from build123d import *

# Parameters (mm, degrees)
SURFACE_EXTRUDE1_1_DEPTH = 1200
THICKEN1_T1              = 3
BOSS_EXTRUDE1_REACH      = 1246.822
SKETCH2_W                = 29.7
SKETCH2_H                = 2


with BuildPart() as body_1:
    # Surface-Extrude1: a surface, the sketch's curves swept straight by 1200 mm
    with BuildLine(Plane.XY, mode=Mode.PRIVATE) as surface_extrude1_1_path:
        Line((-30, 329.67), (-30, 130.766968306))
        ThreePointArc((-30, 130.766968306), (-22.403830344, 63.684928981), (0, 0))
    surface_extrude1_1 = Shell.extrude(surface_extrude1_1_path.wire(), (0 * SURFACE_EXTRUDE1_1_DEPTH, 0 * SURFACE_EXTRUDE1_1_DEPTH, 1 * SURFACE_EXTRUDE1_1_DEPTH))
    add(Solid.thicken(surface_extrude1_1, THICKEN1_T1))

    # Sketch2 → Boss-Extrude1 (add, up to next)
    with BuildSketch(Plane(origin=(0, 329.67, 0), x_dir=(1, 0, 0), z_dir=(0, 1, 0)), mode=Mode.PRIVATE) as boss_extrude1_sk1:
        with Locations((-12.15, -1175)):
            Rectangle(SKETCH2_W, SKETCH2_H)
    boss_extrude1_tool1 = extrude(boss_extrude1_sk1.sketch, amount=-BOSS_EXTRUDE1_REACH, mode=Mode.PRIVATE) - body_1.part
    # Sketch2 → Boss-Extrude1 (add, up to next)
    with BuildSketch(Plane(origin=(0, 329.67, 0), x_dir=(1, 0, 0), z_dir=(0, 1, 0)), mode=Mode.PRIVATE) as boss_extrude1_sk2:
        with Locations((-12.15, -600)):
            Rectangle(SKETCH2_W, SKETCH2_H)
    boss_extrude1_tool2 = extrude(boss_extrude1_sk2.sketch, amount=-BOSS_EXTRUDE1_REACH, mode=Mode.PRIVATE) - body_1.part
    # Sketch2 → Boss-Extrude1 (add, up to next)
    with BuildSketch(Plane(origin=(0, 329.67, 0), x_dir=(1, 0, 0), z_dir=(0, 1, 0)), mode=Mode.PRIVATE) as boss_extrude1_sk3:
        with Locations((-12.15, -25)):
            Rectangle(SKETCH2_W, SKETCH2_H)
    boss_extrude1_tool3 = extrude(boss_extrude1_sk3.sketch, amount=-BOSS_EXTRUDE1_REACH, mode=Mode.PRIVATE) - body_1.part
    add(boss_extrude1_tool1.solids().sort_by_distance((-12.15, 329.67, 1175))[0])
    add(boss_extrude1_tool2.solids().sort_by_distance((-12.15, 329.67, 600))[0])
    add(boss_extrude1_tool3.solids().sort_by_distance((-12.15, 329.67, 25))[0])


solid = body_1.part
Could you check a few things on this model? Use its own coordinates, in mm. A direction names the side the tool comes from. Coordinates: 2 decimals unless noted, no trailing zeros. Order: outer loops, then holes, each group sorted by start corner. A loop starts at its lowest first (then second) coordinate and runs counter-clockwise, first axis right, second up. Notation, with made-up numbers: (-28.5, 71) - (29.5, 71) arc R21 cw to (29.5, 88) - close; hole circle Ø5 at (27, -33). An arc over 180 degrees is marked (long way). Answer in a Markdown table with one row per item. Add a question column.
(1) Will these pins go through, and if not, where does the flat tip stop? pin 1 (15 mm diameter, centred on x = -7.5, y = 110, fed in from -Z); pin 2 (3 mm diameter, centred on x = -2.5, z = 552.5, fed in from -Y); pin 3 (12 mm diameter, centred on y = 192.5, z = 1188.5, fed in from +X).
(2) If we section it at C-C, the plane x = -13: Please give me the cut outline in (y, z).
(3) If we section it at A-A, the plane y = 147: Please give me the cut outline in (x, z).
(4) I need wall thicknesses on L1, parallel to Z at x = -17, y = 102.5; L2, parallel to X at y = 242, z = 136; L3, parallel to X at y = 120.5, z = 274. Which ranges of each line are inside material? Lowest first, please.
(5) If we mould it in two halves opening along Z, with no side actions, what happens to faces 6 (the face through (-28, 329.67, 775)), 7 (the face through (-12, 168, 1174)), 8 (the face through (-19.69, 65.27, 883.49)), 9 (the face through (-12, 168, 24))? For each: released by +Z, released by -Z, zero draft, split by the parting line, or undercut.
(6) On a 3-axis mill with a long thin cutter (end or side, diameter ignored), from which of +Z, -Z, +X, -X, +Y, -Y can I reach the whole of each face in a straight line? I mean faces 1 (the face through (-28, 178, 1200)), 2 (the face through (-12, 168, 601)), 3 (the face through (-28, 178, 0)), 4 (the face through (-27, 232, 12)), 5 (the face through (-27, 232, 1188)). Say none if no direction works.
(7) If we section it at B-B, the plane z = 971: Please give me the cut outline in (x, y), then the cut area to 3 significant figures.
Results are:
| question | item | result |
|---|---|---|
| 1 | pin 1 | stops at z = 24 |
| 1 | pin 2 | stops at y = 2.09 |
| 1 | pin 3 | stops at x = -27 |
| 2 | outline | (31.21, 0) - (40.66, 0) - (40.66, 24) - (329.67, 24) - (329.67, 26) - (40.66, 26) - (40.66, 599) - (329.67, 599) - (329.67, 601) - (40.66, 601) - (40.66, 1174) - (329.67, 1174) - (329.67, 1176) - (40.66, 1176) - (40.66, 1200) - (31.21, 1200) - close |
| 3 | outline | (-30, 0) - (-27, 0) - (-27, 24) - (2.7, 24) - (2.7, 26) - (-27, 26) - (-27, 599) - (2.7, 599) - (2.7, 601) - (-27, 601) - (-27, 1174) - (2.7, 1174) - (2.7, 1176) - (-27, 1176) - (-27, 1200) - (-30, 1200) - close |
| 4 | L1 | z = 24 to 26, 599 to 601, 1174 to 1176 |
| 4 | L2 | x = -30 to -27 |
| 4 | L3 | x = -29.82 to -26.82 |
| 5 | face 6 | zero draft |
| 5 | face 7 | undercut |
| 5 | face 8 | undercut |
| 5 | face 9 | released by -Z |
| 6 | face 1 | +Z, +X, -X, +Y, -Y |
| 6 | face 2 | +X, +Y |
| 6 | face 3 | -Z, +X, -X, +Y, -Y |
| 6 | face 4 | -Z, +X, +Y |
| 6 | face 5 | +Z, +X, +Y |
| 7 | outline | (-30, 130.77) arc R300 ccw to (0, 0) - (2.7, 1.31) arc R297 cw to (-27, 130.77) - (-27, 329.67) - (-30, 329.67) - close |
| 7 | area | 1,000 mm2 |
